Read the model definition and answer for the solid it produces. Units are mm, in the model's axes. Coordinates: 2 decimals unless noted, no trailing zeros. Loops run counter-clockwise (first coordinate to the right, second up) from the corner with the lowest first, then second, coordinate; pieces in that order, holes last. Notation, with made-up numbers: (10.25, 65.25) -> (62.25, 65.25) arc R21 cw to (62.25, 79.25) -> close; hole circle Ø3 at (17, 73). An arc over 180 degrees is marked (long way). Answer as a JSON object with one key per item and string values. Group by question number.
1) Consider probe 1 along Y at (x, z) = (0, 2.5); probe 2 along X at (y, z) = (0.5, 2.25); probe 3 along Y at (x, z) = (1.5, 2.5). Determine where each line is inside the solid, lowest interval first. Write a range as [from, to].
2) Section C-C, the plane z = 2.75 is taken. Give the vertices of the cut face in (x, y).
3) Section A-A, the plane y = 0 is taken. Give the vertices of the cut face in (x, z), plus the area to 3 significant figures.
4) Flat-ended cylindrical pins translate along their axes: P1, Ø1.5, axis at y = -2.5, z = 6.5, coming from the +X side; P2, Ø2.5, axis at x = 0, y = 0, coming from the +Z side. Find the tip coordinate at first contact, or state that the pin passes through.
5) Determine the mould class of faces 1 (the face through (-0.86, -3.874, 3.919)), 2 (the face through (2, -2, 0)), 3 (the face through (-1.8, 0.6, 3.9)) for opening direction X: released by +X, released by -X, zero draft, split by the parting line, or undercut.
from build123d import *

# Parameters (mm, degrees)
SKETCH1_R              = 3.96875
EXTRUDE1_DEPTH         = 7.9375
CHAMFER1_SIZE          = 0.396875
F_10_24_TAPPED_HOLE1_D = 3.7973


with BuildPart() as part:
    # Sketch1 → Extrude1 (new body)
    with BuildSketch(Plane.XY):
        Circle(SKETCH1_R)
    extrude(amount=EXTRUDE1_DEPTH)

    # Chamfer1
    chamfer1_edges = [part.edges().sort_by_distance(p)[0] for p in [
        (-3.96875, 0, 0),
        (-3.96875, 0, 7.9375),
    ]]
    chamfer(chamfer1_edges, length=CHAMFER1_SIZE)

    # #10-24 Tapped Hole1 (through all)
    with Locations(Plane.XY.offset(7.9375)):
        with Locations((0, 0)):
            Hole(F_10_24_TAPPED_HOLE1_D / 2)


solid = part.part
Determined:
{
 "1": {"probe 1": "[-3.97, -1.9], [1.9, 3.97]", "probe 2": "[-3.94, -1.83], [1.83, 3.94]", "probe 3": "[-3.67, -1.16], [1.16, 3.67]"},
 "2": {"outline": "circle Ø7.94 at (0, 0); hole circle Ø3.8 at (0, 0)"},
 "3": {"outline": "(-3.97, 0.4) -> (-3.57, 0) -> (-1.9, 0) -> (-1.9, 7.94) -> (-3.57, 7.94) -> (-3.97, 7.54) -> close; (1.9, 0) -> (3.57, 0) -> (3.97, 0.4) -> (3.97, 7.54) -> (3.57, 7.94) -> (1.9, 7.94) -> close", "area": "32.5 mm²"},
 "4": {"P1": "x = 3.56", "P2": "through"},
 "5": {"face 1": "split by the parting line", "face 2": "zero draft", "face 3": "undercut"}
}
